Work out the finished part from the listing and answer in its coordinate system (mm). Face numbers are marked on the shaded views. A direction names the side the tool comes from. Round coordinates to 2 decimals unless told otherwise and drop trailing zeros. Write each loop counter-clockwise with the first axis right and the second up, starting at its lowest first coordinate (ties: lowest second). Pieces come first, ordered by that corner, then holes.
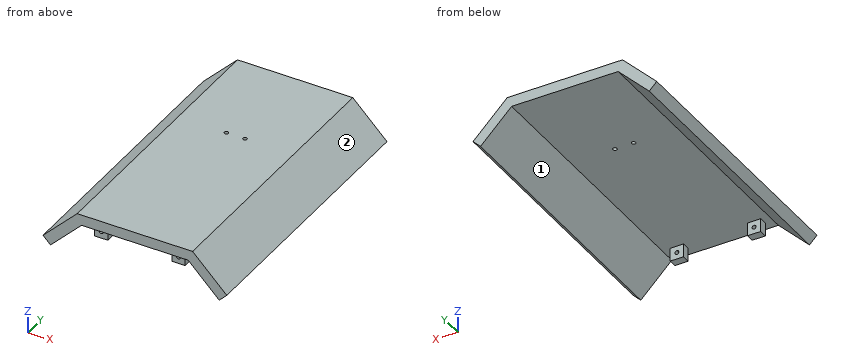
from build123d import *

# Parameters (mm, degrees)
SALIENTE_EXTRUIR1_DEPTH = 206
CROQUIS2_W              = 10
CROQUIS2_H              = 6
SALIENTE_EXTRUIR2_DEPTH = 10
CORTAR_EXTRUIR1_DEPTH   = 10
CROQUIS4_R              = 1.5
CORTAR_EXTRUIR4_DEPTH   = 10


with BuildPart() as part:
    # Croquis1 → Saliente-Extruir1 (new body)
    with BuildSketch(Plane(origin=(0, 0, 0), x_dir=(1, 0, 0), z_dir=(0, 1, 0))):
        Polygon((-40, 0), (40, 0), (63.334523779, 23.334523779), (68.991378029, 17.67766953), (43.313708499, -8), (-43.313708499, -8), (-68.991378029, 17.67766953), (-63.334523779, 23.334523779), align=None)
    extrude(amount=SALIENTE_EXTRUIR1_DEPTH)

    # Croquis2 → Saliente-Extruir2 (add)
    with BuildSketch(Plane(origin=(0, 0, 0), x_dir=(-1, 0, 0), z_dir=(0, 0, -1))):
        with Locations((29, 9.404106992)):
            Rectangle(CROQUIS2_W, CROQUIS2_H)
        with Locations((-29, 9.404106992)):
            Rectangle(CROQUIS2_W, CROQUIS2_H)
    extrude(amount=SALIENTE_EXTRUIR2_DEPTH)

    # Croquis3 → Cortar-Extruir1 (cut)
    with BuildSketch(Plane.XZ.offset(-6.404106992)):
        with BuildLine():
            ThreePointArc((-27.5, -5), (-28.425974851, -3.614180701), (-30.060660172, -3.939339828))
            Line((-30.060660172, -3.939339828), (-27.939339828, -6.060660172))
            ThreePointArc((-27.939339828, -6.060660172), (-27.614180701, -5.574025149), (-27.5, -5))
        make_face()
        with BuildLine():
            Line((-27.939339828, -6.060660172), (-30.060660172, -3.939339828))
            ThreePointArc((-30.060660172, -3.939339828), (-30.060660172, -6.060660172), (-27.939339828, -6.060660172))
        make_face()
        with BuildLine():
            ThreePointArc((29, -3.5), (27.5, -5), (29, -6.5))
            Line((29, -6.5), (29, -3.5))
        make_face()
        with BuildLine():
            Line((29, -3.5), (29, -6.5))
            ThreePointArc((29, -6.5), (30.060660172, -6.060660172), (30.5, -5))
            ThreePointArc((30.5, -5), (30.060660172, -3.939339828), (29, -3.5))
        make_face()
    extrude(amount=-CORTAR_EXTRUIR1_DEPTH, mode=Mode.SUBTRACT)

    # Croquis4 → Cortar-Extruir4 (cut)
    with BuildSketch(Plane.XY.offset(8)):
        with Locations((-7.000068571, 129.596)):
            Circle(CROQUIS4_R)
        with Locations((6.999931429, 129.596)):
            Circle(CROQUIS4_R)
    extrude(amount=-CORTAR_EXTRUIR4_DEPTH, mode=Mode.SUBTRACT)


solid = part.part
Q1. Find section D-D (x = 54). Determine the outline of the cut face in (y, z).
Q2. Given pin 1 (3 mm diameter, centred on y = 8.5, z = -3.5, fed in from -X); pin 2 (8 mm diameter, centred on x = -28.5, z = -4.5, fed in from +Y); pin 3 (1.8 mm diameter, centred on x = 26.5, y = 8, fed in from -Z); pin 4 (12 mm diameter, centred on x = -18, z = -15, fed in from -Y), each flat-ended and moving along its own axis, determine where each tip first touches the part or whether it passes through.
Q3. Find section A-A (y = 70). Determine the outline of the cut face in (x, z), plus the area to 3 significant figures.
Q4. Find section C-C (x = 2). Determine the outline of the cut face in (y, z), plus the area to 3 significant figures.
Q5. Find section B-B (z = 3.5). Determine the outline of the cut face in (x, y), plus the area to 3 significant figures.
Q6. Find the intervals of material crossed by L1, parallel to Z at x = -40, y = 72; L2, parallel to X at y = 35, z = -15; L3, parallel to X at y = 42.5, z = -2.5, in increasing order.
Q7. A tool of negligible diameter and unlimited length cuts with its end or side. For the marked faces 1 and 2, from which of +Z, -Z, +X, -X, +Y, -Y can it reach the whole face along a straight path? Write none if from no direction.
Report:
1. outline: (0, -14) - (206, -14) - (206, -2.69) - (0, -2.69) - close
2. pin 1: stops at x = -56.31
2. pin 2: stops at y = 12.4
2. pin 3: stops at z = -10
2. pin 4: passes through
3. outline: (-68.99, -17.68) - (-63.33, -23.33) - (-40, 0) - (40, 0) - (63.33, -23.33) - (68.99, -17.68) - (43.31, 8) - (-43.31, 8) - close
3. area: 1,220 mm2
4. outline: (0, 0) - (206, 0) - (206, 8) - (0, 8) - close
4. area: 1,650 mm2
5. outline: (-47.81, 0) - (47.81, 0) - (47.81, 206) - (-47.81, 206) - close; hole circle Ø3 at (-7, 129.6); hole circle Ø3 at (7, 129.6)
5. area: 19,700 mm2
6. L1: z = 0 to 8
6. L2: x = -66.31 to -55, 55 to 66.31
6. L3: x = -53.81 to -42.5, 42.5 to 53.81
7. face 1: -Z, +Y, -Y
7. face 2: +Z, +X, +Y, -Y
